Can you work these out from the model? Positions are in its coordinate system, mm. A direction names the side the tool comes from. Round coordinates to 2 decimals unless told otherwise and drop trailing zeros. Write each loop counter-clockwise with the first axis right and the second up, starting at its lowest first coordinate (ties: lowest second). Pieces come first, ordered by that corner, then holes. Notation, with made-up numbers: (-8.75, -13.5) - (13.25, -13.5) arc R17 cw to (13.25, 12.5) - close; hole circle Ø4 at (7, 10). An arc over 180 degrees is marked (long way). One line per item, written item: value. Start each with the question number.
(1) On a 3-axis mill with a long thin cutter (end or side, diameter ignored), from which of +Z, -Z, +X, -X, +Y, -Y can I reach the whole of each face in a straight line? I mean faces 1 (the face through (-14, 10, 8)), 2 (the face through (-4.1, -0.9, 9)), 3 (the face through (10, 4.4, 5.1)), 4 (the face through (-3, 6, 11)), 5 (the face through (13, 11, 2.5)). Say none if no direction works.
(2) Thinking about a two-plate mould opening in Z: for faces 6 (the face through (11, 3, 0)), 7 (the face through (10, -2.5, 0)), 8 (the face through (-2, 6, -11)), which applies, +Z half, -Z half, draft (parallel to the pull), parting line (faces both ways), or undercut?
(3) I want a section at A-A on x = 1. List the corners of the cut face in (y, z) for me.
(4) I want a section at C-C on y = 0. List the corners of the cut face in (x, z) for me, plus the area to 3 significant figures.
(5) I want a section at B-B on z = 0. List the corners of the cut face in (x, y) for me, plus the area to 3 significant figures.
(6) I want a section at D-D on z = 8.5. List the corners of the cut face in (x, y) for me, plus the area to 3 significant figures.
(7) I'm going to push flat-ended pins straight in: pin 1 Ø4 at (x, z) = (0.5, -16) entering from -Y; pin 2 Ø5 at (y, z) = (-1.5, -7) entering from +X; pin 3 Ø6 at (y, z) = (3.5, 6) entering from -X; pin 4 Ø2.5 at (x, z) = (-16, -8.5) entering from -Y. Where does each tip first touch, or does it pass through?
(8) If I drill on L1, parallel to Y at x = 1, z = 16.25; L2, parallel to Z at x = -4, y = 2; L3, parallel to X at y = 0, z = -9.6, over which ranges is the centre line in solid material (lowest first)? Write a range as from..to.
from build123d import *

# Parameters (mm, degrees)
SKETCH1_W               = 22
SKETCH1_H               = 22
BOSS_EXTRUDE1_DEPTH     = 10
SHELL1_T                = -2
SKETCH2_R               = 1.5
SKETCH2_W               = 15
SKETCH2_H               = 7.5
CUT_EXTRUDE1_DEPTH      = 8
SKETCH3_R               = 2.55
CUT_EXTRUDE2_DEPTH      = 8
CUT_EXTRUDE3_DEPTH      = 27.551836095
CUT_EXTRUDE3_DEPTH_BACK = 27.551836095
SKETCH4_R               = 5
BOSS_EXTRUDE2_START     = 10.5
SKETCH5_R               = 6
SKETCH5_R_2             = 5
BOSS_EXTRUDE2_DEPTH     = 10
SKETCH7_R               = 1.5
BOSS_EXTRUDE3_DEPTH     = 2


with BuildPart() as part:
    # Sketch1 → Boss-Extrude1 (new, symmetric)
    with BuildSketch(Plane(origin=(0, 0, 0), x_dir=(1, 0, 0), z_dir=(0, 1, 0))):
        Rectangle(SKETCH1_W, SKETCH1_H)
    extrude(amount=BOSS_EXTRUDE1_DEPTH, both=True)

    # Shell1
    shell1_openings = [part.faces().sort_by_distance(p)[0] for p in [
        (0, -10, 0),
    ]]
    offset(amount=SHELL1_T, openings=shell1_openings, kind=Kind.INTERSECTION)

    # Sketch2 → Cut-Extrude1 (cut)
    with BuildSketch(Plane(origin=(11, 0, 0), x_dir=(0, 0, -1), z_dir=(1, 0, 0))):
        with Locations((-6.475, 5)):
            Circle(SKETCH2_R)
        with Locations(Location((6.475, 5, 0), (0, 0, 180))):
            Circle(SKETCH2_R)
        with Locations((0, -6.25)):
            Rectangle(SKETCH2_W, SKETCH2_H)
    extrude(amount=-CUT_EXTRUDE1_DEPTH, mode=Mode.SUBTRACT)

    # Sketch3 → Cut-Extrude2 (cut)
    with BuildSketch(Plane.ZY.offset(11)):
        Circle(SKETCH3_R)
    extrude(amount=-CUT_EXTRUDE2_DEPTH, mode=Mode.SUBTRACT)

    # Sketch4 → Cut-Extrude3 (cut, two sides: drawn at the far end of the back side and taken through both)
    with BuildSketch(Plane(origin=(0, 0, -11), x_dir=(-1, 0, 0), z_dir=(0, 0, -1)).offset(-CUT_EXTRUDE3_DEPTH_BACK)):
        with Locations((-1, 0)):
            Circle(SKETCH4_R)
    extrude(amount=CUT_EXTRUDE3_DEPTH + CUT_EXTRUDE3_DEPTH_BACK, mode=Mode.SUBTRACT)

    # Sketch5 → Boss-Extrude2 (add)
    with BuildSketch(Plane.XY.offset(BOSS_EXTRUDE2_START)):
        with Locations(Location((1, 0, 0), (0, 0, 180))):
            Circle(SKETCH5_R)
        with Locations(Location((1, 0, 0), (0, 0, 180))):
            Circle(SKETCH5_R_2, mode=Mode.SUBTRACT)
    boss_extrude2 = extrude(amount=BOSS_EXTRUDE2_DEPTH)

    # Mirror4: Boss-Extrude2 across plane
    add(boss_extrude2.mirror(Plane.XY))

    # Sketch7 → Boss-Extrude3 (add)
    with BuildSketch(Plane(origin=(0, 10, 0), x_dir=(1, 0, 0), z_dir=(0, 1, 0))):
        with BuildLine():
            Line((-11, -6), (-16, -6))
            ThreePointArc((-16, -6), (-18.5, -8.5), (-16, -11))
            Line((-16, -11), (-11, -11))
            Line((-11, -11), (11, -11))
            Line((11, -11), (11, -2.5))
            Line((11, -2.5), (16, -2.5))
            ThreePointArc((16, -2.5), (18.5, 0), (16, 2.5))
            Line((16, 2.5), (11, 2.5))
            Line((11, 2.5), (11, 11))
            Line((11, 11), (-11, 11))
            Line((-11, 11), (-16, 11))
            ThreePointArc((-16, 11), (-18.5, 8.5), (-16, 6))
            Line((-16, 6), (-11, 6))
            Line((-11, 6), (-11, -6))
        make_face()
        with Locations(Location((-16, -8.5, 0), (0, 0, 270))):
            Circle(SKETCH7_R, mode=Mode.SUBTRACT)
        with Locations(Location((-16, 8.5, 0), (0, 0, 90))):
            Circle(SKETCH7_R, mode=Mode.SUBTRACT)
        with Locations(Location((16, 0, 0), (0, 0, 270))):
            Circle(SKETCH7_R, mode=Mode.SUBTRACT)
    extrude(amount=BOSS_EXTRUDE3_DEPTH)


solid = part.part
Established:
1. face 1: +Z, -Z, -X, -Y
1. face 2: -Y
1. face 3: +X
1. face 4: +Z
1. face 5: +Z, +X, +Y, -Y
2. face 6: draft
2. face 7: undercut
2. face 8: -Z half
3. outline: (-10, -11) - (-6, -11) - (-6, -20.5) - (-5, -20.5) - (-5, -9) - (-10, -9) - close; (-10, 9) - (-5, 9) - (-5, 20.5) - (-6, 20.5) - (-6, 11) - (-10, 11) - close; (5, -20.5) - (6, -20.5) - (6, -11) - (12, -11) - (12, 11) - (6, 11) - (6, 20.5) - (5, 20.5) - (5, 9) - (8, 9) - (8, -9) - (5, -9) - close
4. outline: (-11, -11) - (-5, -11) - (-5, -20.5) - (-4, -20.5) - (-4, -9) - (-9, -9) - (-9, -2.55) - (-11, -2.55) - close; (-11, 2.55) - (-9, 2.55) - (-9, 9) - (-4, 9) - (-4, 20.5) - (-5, 20.5) - (-5, 11) - (-11, 11) - close; (6, -20.5) - (7, -20.5) - (7, -11) - (11, -11) - (11, 11) - (7, 11) - (7, 20.5) - (6, 20.5) - (6, 9) - (9, 9) - (9, -9) - (6, -9) - close
4. area: 148 mm2
5. outline: (-11, -10) - (-9, -10) - (-9, -2.55) - (-11, -2.55) - close; (-11, 2.55) - (-9, 2.55) - (-9, 8) - (9, 8) - (9, -2.5) - (11, -2.5) - (11, 10) - (14.5, 10) - (14.5, 12) - (-11, 12) - close; (17.5, 10) - (18.5, 10) - (18.5, 12) - (17.5, 12) - close
5. area: 144 mm2
6. outline: (-18.5, 10) - (-17.5, 10) - (-17.5, 12) - (-18.5, 12) - close; (-14.5, 10) - (-11, 10) - (-11, -10) - (-9, -10) - (-9, 8) - (9, 8) - (9, -10) - (11, -10) - (11, 12) - (-14.5, 12) - close
6. area: 169 mm2
7. pin 1: y = -6
7. pin 2: x = 11
7. pin 3: x = -11
7. pin 4: through
8. L1: -6..-5, 5..6
8. L2: -20.5..-9, 9..20.5
8. L3: -11..-4, 6..11
